CAD build for the part. Positions are in the model's coordinates, mm. Round coordinates to 2 decimals unless told otherwise and drop trailing zeros. Order: outer loops, then holes, each group sorted by start corner. A loop starts at its lowest first (then second) coordinate and runs counter-clockwise, first axis right, second up.
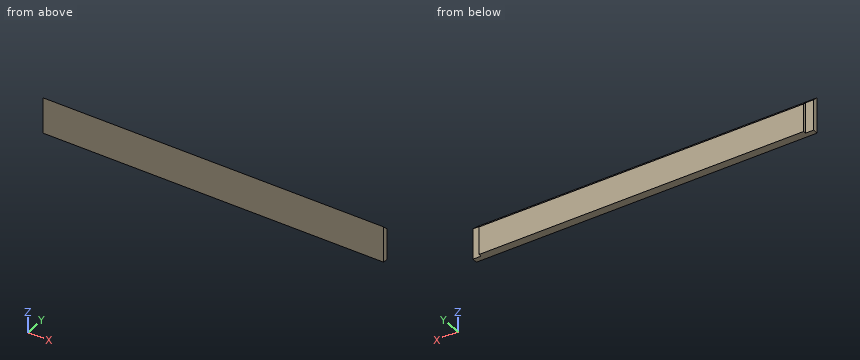
```python
from build123d import *

# Parameters (mm, degrees)
SKETCH_1_W          = 118.3
SKETCH_1_H          = 12.7
EXTRUDE_1_DEPTH     = 2.8
SKETCH_2_W          = 2.8
SKETCH_2_H          = 12.7
CUT_EXTRUDE_1_DEPTH = 1
CUT_EXTRUDE_2_DEPTH = 120.692278835


with BuildPart() as part:
    # 草图1 → 凸台-拉伸1 (new body)
    with BuildSketch(Plane(origin=(0, 0, 0), x_dir=(1, 0, 0), z_dir=(0, 1, 0))):
        with Locations((26.798571429, 11.636428571)):
            Rectangle(SKETCH_1_W, SKETCH_1_H)
    extrude(amount=EXTRUDE_1_DEPTH)

    # 草图2 → 切除-拉伸1 (cut)
    with BuildSketch(Plane(origin=(0, 2.8, 0), x_dir=(1, 0, 0), z_dir=(0, 1, 0))):
        with Locations((-30.951428571, 11.636428571)):
            Rectangle(SKETCH_2_W, SKETCH_2_H)
        with Locations((84.548571429, 11.636428571)):
            Rectangle(SKETCH_2_W, SKETCH_2_H)
    extrude(amount=-CUT_EXTRUDE_1_DEPTH, mode=Mode.SUBTRACT)

    # 草图3 → 切除-拉伸2 (cut, through all)
    with BuildSketch(Plane(origin=(85.948571429, 0, 0), x_dir=(0, 0, -1), z_dir=(1, 0, 0))):
        Polygon((5.286428571, 0), (5.286428571, 2.8), (8.086428571, 2.8), align=None)
    extrude(amount=-CUT_EXTRUDE_2_DEPTH, mode=Mode.SUBTRACT)


solid = part.part
```
1. Drill centre lines: line 1 (X direction, y = 2.15, z = -12.25); line 2 (Z direction, x = 73.5, y = 1.5); line 3 (Z direction, x = 45, y = 1.2). Where is each one in solid material? Low to high.
2. Cut at C-C, the plane y = 1.25. Write the cut outline in (x, z).
3. Pin check, flat tips, straight feed: P1, Ø1.1, axis at y = 2, z = -13, coming from the -X side; P2, Ø1.4, axis at x = 84, z = -12.5, coming from the +Y side; P3, Ø1.1, axis at y = 2.5, z = -10, coming from the +X side. Stop position of each tip, or through.
4. Cut at A-A, the plane z = -16.75. Write the cut outline in (x, y).
5. Cut at B-B, the plane x = 78. Write the cut outline in (y, z).
Outcome:
1. line 1: x = -29.55 to 83.15
1. line 2: z = -17.99 to -6.79
1. line 3: z = -17.99 to -6.49
2. outline: (-32.35, -17.99) - (85.95, -17.99) - (85.95, -6.54) - (-32.35, -6.54) - close
3. P1: stops at x = -32.35
3. P2: stops at y = 1.8
3. P3: stops at x = 83.15
4. outline: (-32.35, 0) - (85.95, 0) - (85.95, 1.8) - (83.15, 1.8) - (83.15, 2.8) - (-29.55, 2.8) - (-29.55, 1.8) - (-32.35, 1.8) - close
5. outline: (0, -17.99) - (2.8, -17.99) - (2.8, -8.09) - (0, -5.29) - close
